Autodesk Fusion 360 part; units mm, degrees
sketch "Sketch1" plane through (0, 0, 0) normal (0, 0, 1) x (1, 0, 0)
  line L0 (0, 0) -> (145, 0)
  line L1 (145, 0) -> (145, 247.018)
  line L2 (145, 247.018) -> (0, 247.018)
  line L3 (0, 247.018) -> (0, 0)
  dimension "d1" = 247.018
  dimension "d2" = 145
extrude "Extrude1" add sketch "Sketch1" along normal blind 3
chamfer "Chamfer1" distance 15 angle 45 2 edges at (0, 0, 1.5) (145, 0, 1.5)
chamfer "Chamfer2" distance 25 angle 45 2 edges at (0, 247.018, 1.5) (145, 247.018, 1.5)
sketch "Sketch3" plane through (0, 0, 3) normal (0, 0, 1) x (-1, 0, 0)
  line L0 (-145, -222.018) -> (-120, -247.018)
  line L1 (-120, -247.018) -> (-25, -247.018)
  line L2 (-25, -247.018) -> (0, -222.018)
  line L3 (0, -222.018) -> (0, -15)
  line L4 (0, -15) -> (-15, 0)
  line L5 (-15, 0) -> (-130, 0)
  line L6 (-130, 0) -> (-145, -15)
  line L7 (-145, -15) -> (-145, -222.018)
  circle A0 centre (-35, -235.018) radius 2.5
  circle A1 centre (-110, -235.018) radius 2.5
  circle A2 centre (-110, -5) radius 2.5
  circle A3 centre (-35, -5) radius 2.5
  circle A4 centre (-35, -5) radius 1.65
  circle A5 centre (-110, -5) radius 1.65
  circle A6 centre (-110, -235.018) radius 1.65
  circle A7 centre (-35, -235.018) radius 1.65
  dimension "d27" = 35
  dimension "d28" = 35
  dimension "d29" = 12
  dimension "d30" = 5
  dimension "d31" = 5
  dimension "d32" = 5
  dimension "d33" = 5
  dimension "d34" = 5
  dimension "d35" = 3.3
  dimension "d36" = 3.3
  dimension "d37" = 3.3
  dimension "d38" = 3.3
extrude "Extrude5" cut sketch "Sketch3" against normal blind 2 contours A0 | A1 | A2 | A3
extrude "Extrude4" cut sketch "Sketch3" against normal blind 3 contours A4 | A5 | A6 | A7
sketch "Sketch4" plane through (0, 0, 3) normal (0, 0, 1) x (-1, 0, 0)
  circle A0 centre (-110, -5) radius 2.5
  circle A1 centre (-110, -235.018) radius 2.5
  circle A2 centre (-35, -5) radius 2.5
  circle A3 centre (-35, -235.018) radius 2.5
  line L0 (-145, -222.018) -> (-120, -247.018)
  line L1 (-120, -247.018) -> (-25, -247.018)
  line L2 (-25, -247.018) -> (0, -222.018)
  line L3 (0, -222.018) -> (0, -15)
  line L4 (0, -15) -> (-15, 0)
  line L5 (-15, 0) -> (-130, 0)
  line L6 (-130, 0) -> (-145, -15)
  line L7 (-145, -15) -> (-145, -222.018)
  line L8 (-72.5, -247.018) -> (-72.5, 0)
  line L9 (0, -118.509) -> (-145, -118.509)
  line L10 (-72.5, -118.509) -> (-72.5, -247.018)
  line L11 (-72.5, -182.7635) -> (0, -182.7635)
  line L12 (-72.5, -118.509) -> (-72.5, 0)
  line L13 (-72.5, -59.2545) -> (0, -59.2545)
  circle A4 centre (-72.5, -182.7635) radius 3.5
  circle A5 centre (-72.5, -59.2545) radius 3.5
  circle A6 centre (-72.5, -53.2545) radius 6
  circle A7 centre (-72.5, -176.7635) radius 6
  dimension "d43" = 7
  dimension "d44" = 7
  dimension "d45" = 12
  dimension "d46" = 12
extrude "Extrude6" cut sketch "Sketch4" against normal blind 3 contours L8 L12 A5 A6 | L8 L12 L13 A5 | L8 L12 A5 A6 | L13 A5 A6 | L8 L12 A5 A6 | L8 L12 A5 A6 | L8 L12 A5 A6
extrude "Extrude7" cut sketch "Sketch4" against normal blind 3 contours L8 L10 A4 A7 | L8 L10 L11 A4 | L8 L10 A4 A7 | L8 L10 A4 A7 | L8 L10 A4 A7 | L11 A4 A7 | L8 L10 A4 A7
extrude "Extrude10" cut sketch "Sketch3" against normal blind 1 contours L0 L1 L2 L3 L4 L5 L6 L7
extrude "Extrude11" cut 1 faces at (122.568, 136.9318, 0) along direction (0, 0, 1) blind 0.5
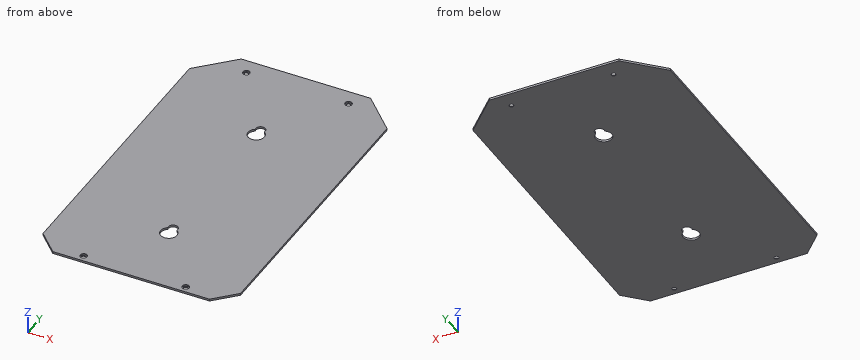
Here's how the part is built. I have some questions about the finished solid (model axes, mm). Give positions to 0.01 mm unless a question says otherwise; leave off trailing zeros. Write each loop counter-clockwise with the first axis right and the second up, starting at its lowest first coordinate (ties: lowest second). Pieces come first, ordered by that corner, then holes.
(1) Imagine slicing it at C-C, the plane x = 12. Write out the boundary of the cut face in (y, z).
Output values:
outline: (3, 0.5) - (234.02, 0.5) - (234.02, 2) - (3, 2) - close
(2) Imagine slicing it at B-B, the plane z = 1.5. Write out the boundary of the cut face in (x, y).
Output values:
outline: (0, 15) - (15, 0) - (130, 0) - (145, 15) - (145, 222.02) - (120, 247.02) - (25, 247.02) - (0, 222.02) - close; hole circle Ø5 at (35, 5); hole circle Ø5 at (35, 235.02); hole (69.15, 58.23) arc R6 ccw (long way) to (75.85, 58.23) arc R3.5 ccw (long way) to start; hole (69.15, 181.74) arc R6 ccw (long way) to (75.85, 181.74) arc R3.5 ccw (long way) to start; hole circle Ø5 at (110, 5); hole circle Ø5 at (110, 235.02)
(3) If I drill on L1, parallel to Y at x = 72.5, z = 1.25; L2, parallel to Y at x = 110, z = 0.8; L3, parallel to X at y = 236, z = 0.6, over which ranges is the centre line in solid material (lowest first)?
Output values:
L1: y = 0 to 47.25, 62.75 to 170.76, 186.26 to 247.02
L2: y = 0 to 3.35, 6.65 to 233.37, 236.67 to 247.02
L3: x = 13.98 to 33.67, 36.33 to 108.67, 111.33 to 131.02
(4) Imagine slicing it at A-A, the plane x = 72.5. Write out the boundary of the cut face in (y, z), and give its area (3 significant figures).
Output values:
outline: (0, 0.5) - (47.25, 0.5) - (47.25, 2) - (0, 2) - close; (62.75, 0.5) - (170.76, 0.5) - (170.76, 2) - (62.75, 2) - close; (186.26, 0.5) - (247.02, 0.5) - (247.02, 2) - (186.26, 2) - close
area: 324 mm2
(5) Will this pin go through, and if not, where does the flat tip stop? pin 1 (1.5 mm diameter, centred on x = 36, y = 235.5, fed in from +Z).
Output values:
pin 1: stops at z = 1
